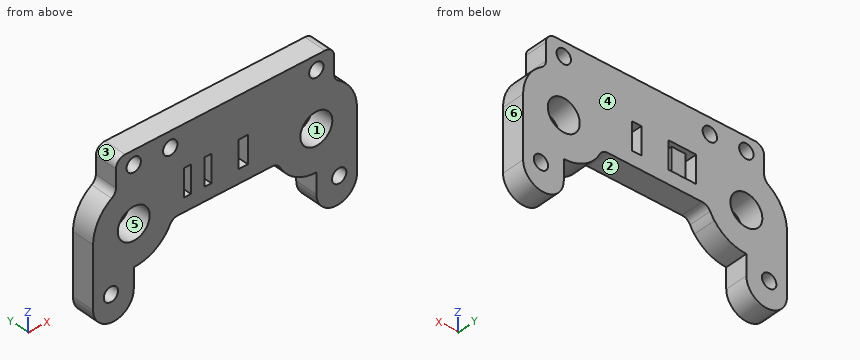
```python
from build123d import *

# Parameters (mm, degrees)
BOSS_EXTRUDE1_DEPTH = 6.35
SKETCH3_R           = 4.445
CUT_EXTRUDE2_DEPTH  = 6.35
SKETCH11_W          = 2.54
SKETCH11_H          = 7.62
SKETCH11_W_2        = 1.905
CUT_EXTRUDE6_DEPTH  = 6.35
SKETCH14_W          = 3.81
SKETCH14_H          = 7.62
CUT_EXTRUDE8_DEPTH  = 1.27
SKETCH8_R           = 2
CUT_EXTRUDE10_DEPTH = 6.35
SKETCH15_R          = 2
CUT_EXTRUDE11_DEPTH = 6.35


with BuildPart() as part:
    # Sketch1 → Boss-Extrude1 (new body)
    with BuildSketch(Plane(origin=(0, 0, 0), x_dir=(1, 0, 0), z_dir=(0, 1, 0))):
        with BuildLine():
            Line((-25.4, 11.309999986), (-25.4, 16.964999979))
            ThreePointArc((-25.4, 16.964999979), (-31.054999993, 22.619999972), (-36.709999986, 16.964999979))
            Line((-36.709999986, 16.964999979), (-36.709999986, 11.309999986))
            Line((-36.709999986, 11.309999986), (-36.709999986, 0))
            ThreePointArc((-36.709999986, 0), (-35.329369206, -5.415138673), (-31.524548724, -9.508207119))
            ThreePointArc((-31.524548724, -9.508207119), (-30.670062071, -10.427428504), (-30.359999986, -11.643560444))
            Line((-30.359999986, -11.643560444), (-30.359999986, -16.51))
            ThreePointArc((-30.359999986, -16.51), (-29.61605121, -18.306051224), (-27.819999986, -19.05))
            Line((-27.819999986, -19.05), (27.819999986, -19.05))
            ThreePointArc((27.819999986, -19.05), (29.61605121, -18.306051224), (30.359999986, -16.51))
            Line((30.359999986, -16.51), (30.359999986, -11.643560444))
            ThreePointArc((30.359999986, -11.643560444), (30.670062071, -10.427428504), (31.524548724, -9.508207119))
            ThreePointArc((31.524548724, -9.508207119), (35.329369206, -5.415138673), (36.709999986, 0))
            Line((36.709999986, 0), (36.709999986, 11.309999986))
            Line((36.709999986, 11.309999986), (36.709999986, 16.964999979))
            ThreePointArc((36.709999986, 16.964999979), (31.054999993, 22.619999972), (25.4, 16.964999979))
            Line((25.4, 16.964999979), (25.4, 11.309999986))
            ThreePointArc((25.4, 11.309999986), (20.457539197, 10.172914081), (16.508889627, 6.990297277))
            ThreePointArc((16.508889627, 6.990297277), (15.885935778, 6.115446153), (15.348771474, 5.185451262))
            ThreePointArc((15.348771474, 5.185451262), (14.413140747, 4.180950232), (13.091466391, 3.81))
            Line((13.091466391, 3.81), (-13.091466391, 3.81))
            ThreePointArc((-13.091466391, 3.81), (-14.413140747, 4.180950232), (-15.348771474, 5.185451262))
            ThreePointArc((-15.348771474, 5.185451262), (-15.885935775, 6.115446149), (-16.508889621, 6.990297269))
            ThreePointArc((-16.508889621, 6.990297269), (-20.457539193, 10.172914079), (-25.4, 11.309999986))
        make_face()
    extrude(amount=BOSS_EXTRUDE1_DEPTH)

    # Sketch3 → Cut-Extrude2 (cut)
    with BuildSketch(Plane(origin=(0, 6.35, 0), x_dir=(1, 0, 0), z_dir=(0, 1, 0))):
        with Locations((-25.4, 0)):
            Circle(SKETCH3_R)
        with Locations((25.4, 0)):
            Circle(SKETCH3_R)
    extrude(amount=-CUT_EXTRUDE2_DEPTH, mode=Mode.SUBTRACT)

    # Sketch11 → Cut-Extrude6 (cut)
    with BuildSketch(Plane(origin=(0, 6.35, 0), x_dir=(1, 0, 0), z_dir=(0, 1, 0))):
        with Locations((5.08, -3.81)):
            Rectangle(SKETCH11_W, SKETCH11_H)
        with Locations((-4.7625, -3.81)):
            Rectangle(SKETCH11_W_2, SKETCH11_H)
        with Locations((-10.4775, -3.81)):
            Rectangle(SKETCH11_W_2, SKETCH11_H)
    extrude(amount=-CUT_EXTRUDE6_DEPTH, mode=Mode.SUBTRACT)

    # Sketch14 → Cut-Extrude8 (cut)
    with BuildSketch(Plane(origin=(0, 6.35, 0), x_dir=(1, 0, 0), z_dir=(0, 1, 0))):
        with Locations((-7.62, -3.81)):
            Rectangle(SKETCH14_W, SKETCH14_H)
    extrude(amount=-CUT_EXTRUDE8_DEPTH, mode=Mode.SUBTRACT)

    # Sketch8 → Cut-Extrude10 (cut)
    with BuildSketch(Plane(origin=(0, 6.35, 0), x_dir=(1, 0, 0), z_dir=(0, 1, 0))):
        with Locations((-31.75, 15.24)):
            Circle(SKETCH8_R)
        with Locations((25.4, -15.24)):
            Circle(SKETCH8_R)
        with Locations((-25.4, -15.24)):
            Circle(SKETCH8_R)
        with Locations((31.75, 15.24)):
            Circle(SKETCH8_R)
    extrude(amount=-CUT_EXTRUDE10_DEPTH, mode=Mode.SUBTRACT)

    # Sketch15 → Cut-Extrude11 (cut)
    with BuildSketch(Plane(origin=(0, 6.35, 0), x_dir=(1, 0, 0), z_dir=(0, 1, 0))):
        with Locations((-15.24, -14.732)):
            Circle(SKETCH15_R)
    extrude(amount=-CUT_EXTRUDE11_DEPTH, mode=Mode.SUBTRACT)


solid = part.part
```
Source: CAD feature listing. Evaluate the final solid. Frame: model axes, mm. Face numbers are marked on the shaded views. A direction names the side the tool comes from. Round coordinates to 2 decimals unless told otherwise and drop trailing zeros. Write each loop counter-clockwise with the first axis right and the second up, starting at its lowest first coordinate (ties: lowest second). Pieces come first, ordered by that corner, then holes. Notation, with made-up numbers: M 26,7.25 L 75,7.25 A13 cw 75,24.25 Z; hole C -14,19.5 d11. An arc over 180 degrees is marked long. Answer as a JSON object with one key per item and string values. Group by question number.
(1) Section query B-B on x = 28.5. Output: boundary loops of the cut face in (y, z).
(2) Ray query, line 1 (X direction, y = 2.5, z = -15.5); line 2 (Z direction, x = 4, y = 3.25); line 3 (X direction, y = 1.25, z = 2) (3 decimals). Return the intervals inside material, ascending. Write a range as [from, to].
(3) Section query A-A on z = -15.24. Output: boundary loops of the cut face in (x, y), then the cut area to 3 significant figures.
(4) Reachability of the marked faces 1 and 2 from +Z, -Z, +X, -X, +Y, -Y: full face, straight path, thin tool, end or side. Return the list, or none.
(5) Section query C-C on y = 2.5. State how many separate pieces and enclosed holes the cut face has, then the cut area to 3 significant figures.
(6) First-contact query: pin 1 (2.5 mm diameter, centred on y = 3.5, z = 14, fed in from -X); pin 2 (3 mm diameter, centred on x = -3, y = 4.5, fed in from -Z); pin 3 (1.1 mm diameter, centred on x = -7.5, z = 5.5, fed in from +Y); pin 4 (12 mm diameter, centred on x = -22.5, z = -0.5, fed in from -Y). Flat tips, straight axial feed; report the tip coordinate or a pass-through.
(7) Mould query, pull axis X, two halves, no side actions, for the marked faces 3, 4, 5 and 6. Classes: +X half, -X half, draft (parallel to the pull), parting line (faces both ways), or undercut.
(8) Section query D-D on x = 17.5. Output: boundary loops of the cut face in (y, z), then the cut area to 3 significant figures.
Computed values:
{
 "1": {"outline": "M 0,-22.01 L 6.35,-22.01 L 6.35,-3.19 L 0,-3.19 Z; M 0,3.19 L 6.35,3.19 L 6.35,18.96 L 0,18.96 Z"},
 "2": {"line 1": "[-36.71, -33.73], [-29.77, -25.4], [25.4, 29.77], [33.73, 36.71]", "line 2": "[-3.81, 0], [7.62, 19.05]", "line 3": "[-36.532, -29.37], [-21.43, -11.43], [-9.525, -5.715], [-3.81, 3.81], [6.35, 21.43], [29.37, 36.532]"},
 "3": {"outline": "M -36.71,0 L -33.75,0 L -33.75,6.35 L -36.71,6.35 Z; M -29.75,0 L -25.4,0 L -25.4,6.35 L -29.75,6.35 Z; M 25.4,0 L 29.75,0 L 29.75,6.35 L 25.4,6.35 Z; M 33.75,0 L 36.71,0 L 36.71,6.35 L 33.75,6.35 Z", "area": "92.8 mm^2"},
 "4": {"face 1": "+Y, -Y", "face 2": "-Z, +Y, -Y"},
 "5": {"separate pieces": "1", "enclosed holes": "10", "area": "1,810 mm^2"},
 "6": {"pin 1": "x = -30.36", "pin 2": "z = -3.81", "pin 3": "y = 5.08", "pin 4": "y = 0"},
 "7": {"face 3": "-X half", "face 4": "draft", "face 5": "undercut", "face 6": "+X half"},
 "8": {"outline": "M 0,-8.09 L 6.35,-8.09 L 6.35,19.05 L 0,19.05 Z", "area": "172 mm^2"}
}
